Work out the finished part from the listing and answer in its coordinate system (mm). Face numbers are marked on the shaded views. Round coordinates to 2 decimals unless told otherwise and drop trailing zeros. Order: outer loops, then holes, each group sorted by start corner. A loop starts at its lowest first (then second) coordinate and runs counter-clockwise, first axis right, second up.
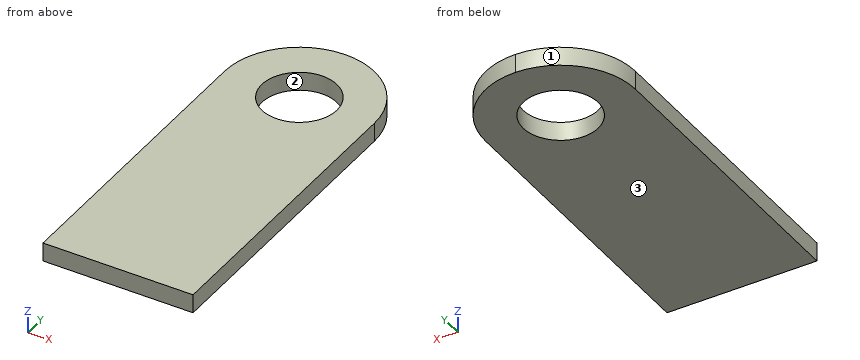
from build123d import *

# Parameters (mm, degrees)
SKETCH1_W           = 4
SKETCH1_H           = 0.5
BOSS_EXTRUDE1_DEPTH = 10
FILLET1_R           = 2
SKETCH2_R           = 1
CUT_EXTRUDE1_DEPTH  = 0.5


with BuildPart() as part:
    # Sketch1 → Boss-Extrude1 (new body)
    with BuildSketch(Plane(origin=(0, 0, 0), x_dir=(1, 0, 0), z_dir=(0, 1, 0))):
        Rectangle(SKETCH1_W, SKETCH1_H)
    extrude(amount=BOSS_EXTRUDE1_DEPTH)

    # Fillet1
    fillet1_edges = [part.edges().sort_by_distance(p)[0] for p in [
        (-2, 10, 0),
        (2, 10, 0),
    ]]
    fillet(fillet1_edges, radius=FILLET1_R - 0.0001)  # a hair under: the kernel refuses the full size

    # Sketch2 → Cut-Extrude1 (cut)
    with BuildSketch(Plane.XY.offset(0.25)):
        with Locations((0, 8)):
            Circle(SKETCH2_R)
    extrude(amount=-CUT_EXTRUDE1_DEPTH, mode=Mode.SUBTRACT)


solid = part.part
Item 1: Find section A-A (x = 0.85). Write down the section's boundary in (y, z), plus the area to 3 significant figures.
Item 2: Find section D-D (x = -1.6). Write down the section's boundary in (y, z).
Item 3: For a pull along Y with two mould halves and no side action, classify the marked faces 1, 2 and 3 as released by +Y, released by -Y, zero draft, split by the parting line, or undercut.
Item 4: Find the intervals of material crossed by line 1 along Y through (x, z) = (0, -0.05); line 2 along Y through (x, z) = (-0.4, -0.15); line 3 along Y through (x, z) = (-1.45, -0.05), in increasing order.
Item 5: Find section C-C (y = 8.5). Write down the section's boundary in (x, z).
Model answer:
1. outline: (0, -0.25) - (7.47, -0.25) - (7.47, 0.25) - (0, 0.25) - close; (8.53, -0.25) - (9.81, -0.25) - (9.81, 0.25) - (8.53, 0.25) - close
1. area: 4.38 mm2
2. outline: (0, -0.25) - (9.2, -0.25) - (9.2, 0.25) - (0, 0.25) - close
3. face 1: released by +Y
3. face 2: undercut
3. face 3: zero draft
4. line 1: y = 0 to 7, 9 to 10
4. line 2: y = 0 to 7.08, 8.92 to 9.96
4. line 3: y = 0 to 9.38
5. outline: (-1.94, -0.25) - (-0.87, -0.25) - (-0.87, 0.25) - (-1.94, 0.25) - close; (0.87, -0.25) - (1.94, -0.25) - (1.94, 0.25) - (0.87, 0.25) - close
